Work out the finished part from the listing and answer in its coordinate system (mm). A direction names the side the tool comes from. Give positions to 0.01 mm unless a question says otherwise; leave off trailing zeros. Write each loop counter-clockwise with the first axis right and the second up, starting at its lowest first coordinate (ties: lowest second). Pieces come first, ordered by that corner, then holes.
1) Straight lines are drawn through the part: probe 1 along Z at (x, y) = (-7.75, -37); probe 2 along X at (y, z) = (-31, -2); probe 3 along X at (y, z) = (-34.5, -0.25). For each, find the intervals that lie inside material, in ascending order.
2) Find section A-A (y = -37.5). Determine the outline of the cut face in (x, z), plus the area to 3 significant figures.
3) Determine the mould class of faces 1 (the face through (-1, -32, -0.38)), 2 (the face through (-15.544, -64.014, 0.325)), 3 (the face through (-15.841, -13.133, -6.299)) for opening direction Y: pulls with the +Y half, pulls with the -Y half, needs draft (parallel to the pull), parting line crosses it, or undercut.
4) Given pin 1 Ø2 at (x, z) = (6, -2) entering from -Y, flat-ended and moving along its own axis, determine where the tip first touches the part or whether it passes through.
5) A tool of negligible diameter and unlimited length cuts with its end or side. For faces 4 (the face through (-15.841, -54.226, -6.299)), 5 (the face through (-14.855, -32, -7)), from which of +Z, -Z, +X, -X, +Y, -Y can it reach the whole face along a straight path? Write none if from no direction.
```python
from build123d import *

# Parameters (mm, degrees)
F1_DEPTH = 65
F2_SIZE  = 1.99999
F3_R     = 1.6
F4_DEPTH = 2


# Not quite as in the source:
# - a fillet or chamfer is up to 0.001 mm smaller than in the source, because OpenCascade refuses the exact size


with BuildPart() as f1:
    # F0 (on Front) → F1 (new body)
    with BuildSketch(Plane.XZ):
        with BuildLine():
            Line((-16.8549300951, -0.3802398592), (-16.8549300951, -13.3802398592))
            Line((-16.8549300951, -13.3802398592), (-14.8549300951, -13.3802398592))
            Line((-14.8549300951, -13.3802398592), (-14.8549300951, -1.3802398592))
            ThreePointArc((-14.8549300951, -1.3802398592), (-14.5620368763, -0.673133078), (-13.8549300951, -0.3802398592))
            Line((-13.8549300951, -0.3802398592), (13.1450699049, -0.3802398592))
            Line((13.1450699049, -0.3802398592), (13.1450699049, 1.6197601408))
            Line((13.1450699049, 1.6197601408), (-14.8549300951, 1.6197601408))
            ThreePointArc((-14.8549300951, 1.6197601408), (-16.2691436574, 1.0339737031), (-16.8549300951, -0.3802398592))
        make_face()
    extrude(amount=F1_DEPTH)

    # F2 (size 2 in the source; OpenCascade refuses exactly that, so slightly less here)
    f2_edges = [f1.edges().sort_by_distance(p)[0] for p in [
        (-16.85493, -65, -6.88024),
    ]]
    chamfer(f2_edges, length=F2_SIZE)

    # F3 (on face) → F4 (cut, through all)
    with BuildSketch(Plane.YZ.offset(-14.8549300951)):
        with Locations((-53.0466809869, -7.3802398592)):
            Circle(F3_R)
        with Locations((-11.9533190131, -7.3802398592)):
            Circle(F3_R)
    extrude(amount=-F4_DEPTH, mode=Mode.SUBTRACT)


solid = f1.part
```
Results:
1. probe 1: z = -0.38 to 1.62
1. probe 2: x = -16.85 to -14.85
1. probe 3: x = -16.85 to 13.15
2. outline: (-16.85, -13.38) - (-14.85, -13.38) - (-14.85, -1.38) arc R1 cw to (-13.85, -0.38) - (13.15, -0.38) - (13.15, 1.62) - (-14.85, 1.62) arc R2 ccw to (-16.85, -0.38) - close
2. area: 85.4 mm2
3. face 1: needs draft
3. face 2: pulls with the -Y half
3. face 3: undercut
4. pin 1: passes through
5. face 4: +X, -X
5. face 5: -Z, +X, +Y, -Y
